from build123d import *

# Parameters (mm, degrees)
SKETCH1_W           = 40
SKETCH1_H           = 29.3
SKETCH1_H_2         = 8.7
BOSS_EXTRUDE1_DEPTH = 20.2
SKETCH2_R           = 2.65
BOSS_EXTRUDE2_DEPTH = 5.2
SKETCH3_W           = 0.446843519
SKETCH3_H           = 1.306192745
SKETCH3_H_2         = 1.306192746
CUT_EXTRUDE1_DEPTH  = 5.2
FILLET1_R           = 3
CHAMFER1_SIZE       = 5
SKETCH4_R           = 6
BOSS_EXTRUDE3_DEPTH = 1
BOSS_EXTRUDE4_DEPTH = 0.5


with BuildPart() as part:
    # Sketch1 → Boss-Extrude1 (new body)
    with BuildSketch(Plane.XY):
        Rectangle(SKETCH1_W, SKETCH1_H)
        Polygon((-27, 14.65), (-20, 14.65), (20, 14.65), (27, 14.65), (27, 17.15), (20, 17.15), (-20, 17.15), (-27, 17.15), align=None)
        with Locations((0, 21.5)):
            Rectangle(SKETCH1_W, SKETCH1_H_2)
    extrude(amount=BOSS_EXTRUDE1_DEPTH)

    # Sketch2 → Boss-Extrude2 (add)
    with BuildSketch(Plane(origin=(0, 25.85, 0), x_dir=(1, 0, 0), z_dir=(0, 1, 0))):
        with Locations((-9.5, -10.1)):
            Circle(SKETCH2_R)
    extrude(amount=BOSS_EXTRUDE2_DEPTH)

    # Sketch3 → Cut-Extrude1 (cut)
    with BuildSketch(Plane(origin=(0, 17.15, 0), x_dir=(1, 0, 0), z_dir=(0, 1, 0))):
        with BuildLine():
            Line((-25.540550997, -5.731244645), (-25.540550997, -4.4250519))
            Line((-25.540550997, -4.4250519), (-25.882669663, -4.4250519))
            ThreePointArc((-25.882669663, -4.4250519), (-25.99986637, -5.076880711), (-25.897769796, -5.731244645))
            Line((-25.897769796, -5.731244645), (-25.540550997, -5.731244645))
        make_face()
        with BuildLine():
            Line((-25.882669663, -4.4250519), (-25.540550997, -4.4250519))
            Line((-25.540550997, -4.4250519), (-25.540550997, -5.731244645))
            Line((-25.540550997, -5.731244645), (-25.897769796, -5.731244645))
            ThreePointArc((-25.897769796, -5.731244645), (-23.680265416, -7.074277031), (-22, -5.1))
            ThreePointArc((-22, -5.1), (-23.657464839, -3.129550898), (-25.882669663, -4.4250519))
        make_face()
        with BuildLine():
            ThreePointArc((-25.897769796, -5.731244645), (-25.99986637, -5.076880711), (-25.882669663, -4.4250519))
            Line((-25.882669663, -4.4250519), (-27.446843519, -4.4250519))
            Line((-27.446843519, -4.4250519), (-27.446843519, -5.731244645))
            Line((-27.446843519, -5.731244645), (-25.897769796, -5.731244645))
        make_face()
        with BuildLine():
            Line((-25.540550997, -15.653096373), (-25.540550997, -14.346903627))
            Line((-25.540550997, -14.346903627), (-25.852794067, -14.346903627))
            ThreePointArc((-25.852794067, -14.346903627), (-25.997198696, -14.994182379), (-25.922000105, -15.653096373))
            Line((-25.922000105, -15.653096373), (-25.540550997, -15.653096373))
        make_face()
        with BuildLine():
            Line((-25.852794067, -14.346903627), (-25.540550997, -14.346903627))
            Line((-25.540550997, -14.346903627), (-25.540550997, -15.653096373))
            Line((-25.540550997, -15.653096373), (-25.922000105, -15.653096373))
            ThreePointArc((-25.922000105, -15.653096373), (-23.720715387, -17.080404026), (-22, -15.1))
            ThreePointArc((-22, -15.1), (-23.616325746, -13.137146448), (-25.852794067, -14.346903627))
        make_face()
        with BuildLine():
            ThreePointArc((-25.922000105, -15.653096373), (-25.997198696, -14.994182379), (-25.852794067, -14.346903627))
            Line((-25.852794067, -14.346903627), (-27.446843519, -14.346903627))
            Line((-27.446843519, -14.346903627), (-27.446843519, -15.653096373))
            Line((-27.446843519, -15.653096373), (-25.922000105, -15.653096373))
        make_face()
        with Locations((27.223421759, -5.078148273)):
            Rectangle(SKETCH3_W, SKETCH3_H)
        with BuildLine():
            ThreePointArc((26, -5.1), (25.974277031, -5.419734584), (25.897769796, -5.731244645))
            Line((25.897769796, -5.731244645), (27, -5.731244645))
            Line((27, -5.731244645), (27, -4.4250519))
            Line((27, -4.4250519), (25.882669663, -4.4250519))
            ThreePointArc((25.882669663, -4.4250519), (25.970449102, -4.757464839), (26, -5.1))
        make_face()
        with BuildLine():
            Line((25.540550997, -4.4250519), (25.540550997, -5.731244645))
            Line((25.540550997, -5.731244645), (25.897769796, -5.731244645))
            ThreePointArc((25.897769796, -5.731244645), (25.974277031, -5.419734584), (26, -5.1))
            ThreePointArc((26, -5.1), (25.970449102, -4.757464839), (25.882669663, -4.4250519))
            Line((25.882669663, -4.4250519), (25.540550997, -4.4250519))
        make_face()
        with BuildLine():
            Line((25.897769796, -5.731244645), (25.540550997, -5.731244645))
            Line((25.540550997, -5.731244645), (25.540550997, -4.4250519))
            Line((25.540550997, -4.4250519), (25.882669663, -4.4250519))
            ThreePointArc((25.882669663, -4.4250519), (22.00013363, -5.123119289), (25.897769796, -5.731244645))
        make_face()
        with Locations((27.223421759, -15)):
            Rectangle(SKETCH3_W, SKETCH3_H_2)
        with BuildLine():
            Line((27, -15.653096373), (27, -14.346903627))
            Line((27, -14.346903627), (25.852794067, -14.346903627))
            ThreePointArc((25.852794067, -14.346903627), (25.962853552, -14.716325746), (26, -15.1))
            ThreePointArc((26, -15.1), (25.980404026, -15.379284613), (25.922000105, -15.653096373))
            Line((25.922000105, -15.653096373), (27, -15.653096373))
        make_face()
        with BuildLine():
            ThreePointArc((26, -15.1), (25.962853552, -14.716325746), (25.852794067, -14.346903627))
            Line((25.852794067, -14.346903627), (25.540550997, -14.346903627))
            Line((25.540550997, -14.346903627), (25.540550997, -15.653096373))
            Line((25.540550997, -15.653096373), (25.922000105, -15.653096373))
            ThreePointArc((25.922000105, -15.653096373), (25.980404026, -15.379284613), (26, -15.1))
        make_face()
        with BuildLine():
            Line((25.540550997, -14.346903627), (25.852794067, -14.346903627))
            ThreePointArc((25.852794067, -14.346903627), (22.002801304, -15.205817621), (25.922000105, -15.653096373))
            Line((25.922000105, -15.653096373), (25.540550997, -15.653096373))
            Line((25.540550997, -15.653096373), (25.540550997, -14.346903627))
        make_face()
    extrude(amount=-CUT_EXTRUDE1_DEPTH, mode=Mode.SUBTRACT)

    # Fillet1
    fillet1_edges = [part.edges().sort_by_distance(p)[0] for p in [
        (-27, 15.9, 0),
        (27, 15.9, 0),
        (27, 15.9, 20.2),
        (-27, 15.9, 20.2),
    ]]
    fillet(fillet1_edges, radius=FILLET1_R)

    # Chamfer1
    chamfer1_edges = [part.edges().sort_by_distance(p)[0] for p in [
        (20, 25.85, 10.1),
    ]]
    chamfer(chamfer1_edges, length=CHAMFER1_SIZE)

    # Sketch4 → Boss-Extrude3 (add)
    with BuildSketch(Plane(origin=(0, 25.85, 0), x_dir=(1, 0, 0), z_dir=(0, 1, 0))):
        with Locations((-9.5, -10.1)):
            Circle(SKETCH4_R)
    extrude(amount=BOSS_EXTRUDE3_DEPTH)

    # Sketch5 → Boss-Extrude4 (add)
    with BuildSketch(Plane(origin=(0, 25.85, 0), x_dir=(1, 0, 0), z_dir=(0, 1, 0))):
        with BuildLine():
            Line((-9.5, -1.789920634), (8.092095239, -1.789920634))
            ThreePointArc((8.092095239, -1.789920634), (9.506308801, -2.375707072), (10.092095239, -3.789920634))
            Line((10.092095239, -3.789920634), (10.092095239, -16.410079366))
            ThreePointArc((10.092095239, -16.410079366), (9.506308801, -17.824292928), (8.092095239, -18.410079366))
            Line((8.092095239, -18.410079366), (-9.5, -18.410079366))
            ThreePointArc((-9.5, -18.410079366), (-17.810079366, -10.1), (-9.5, -1.789920634))
        make_face()
    extrude(amount=BOSS_EXTRUDE4_DEPTH)


solid = part.part
For this review, take the finished solid that the model builds, in its own axes (mm). A direction names the side the tool comes from. Coordinates: 2 decimals unless noted, no trailing zeros. Loops run counter-clockwise (first coordinate to the right, second up) from the corner with the lowest first, then second, coordinate; pieces in that order, holes last. Notation, with made-up numbers: (48.5, -20.5) -> (63.5, -20.5) arc R12 cw to (63.5, -8.5) -> close; hole circle Ø5 at (-35, 69.25). An arc over 180 degrees is marked (long way). Write each question's results on one line, items separated by ' | '.
Q1. Machinability: for faces 1 (the flat face through (-3, 25.85, 1)), 2 (the flat face through (26.4, 15.9, 14.347)), 3 (the flat face through (-24, 14.65, 10)), 4 (the flat face through (-23, 17.15, 10)), 5 (the flat face through (20, 0, 10)), which of the approach directions +Z, -Z, +X, -X, +Y, -Y give a long, thin tool a straight path to every point of the face, cutting with its end or side? Answer none if there is none.
Taken from the geometry:
face 1: +Y | face 2: +X, +Y, -Y | face 3: +Z, -Z, -X, -Y | face 4: +Z, -Z, -X, +Y | face 5: +Z, -Z, +X, -Y
Q2. Add section C-C, the plane x = 16. State the section outline as (y, z) points, then the cut area to 3 significant figures.
Taken from the geometry:
outline: (-14.65, 0) -> (24.85, 0) -> (24.85, 20.2) -> (-14.65, 20.2) -> close | area: 798 mm²
Q3. Add section B-B, the plane y = 9. State the section outline as (x, z) points, then the cut area to 3 significant figures.
Taken from the geometry:
outline: (-20, 0) -> (20, 0) -> (20, 20.2) -> (-20, 20.2) -> close | area: 808 mm²
Q4. To check wall thickness, follow line 1 along Z through (x, y) = (24, 16); line 2 along X through (y, z) = (15.65, 5.1); line 3 along Y through (x, z) = (5.5, 13). State the ranges of each line that lie inside material, in increasing order. Write a range as [from, to].
Taken from the geometry:
line 1: [0, 3.1], [7.1, 13.1], [17.1, 20.2] | line 2: [-22, 22] | line 3: [-14.65, 26.35]
Q5. For pin 1 Ø0.6 at (x, y) = (-26, 15.5) entering from +Z; pin 2 Ø3.5 at (x, z) = (24, 7.5) entering from -Y; pin 3 Ø3.5 at (x, z) = (22.5, 8) entering from +Y, all flat-tipped, find the tip position at first contact; note any pin that passes through.
Taken from the geometry:
pin 1: z = 19.67 | pin 2: y = 14.65 | pin 3: y = 17.15
Q6. Add section A-A, the plane x = -8.5. State the section outline as (y, z) points.
Taken from the geometry:
outline: (-14.65, 0) -> (25.85, 0) -> (25.85, 1.79) -> (26.35, 1.79) -> (26.35, 4.18) -> (26.85, 4.18) -> (26.85, 7.65) -> (31.05, 7.65) -> (31.05, 12.55) -> (26.85, 12.55) -> (26.85, 16.02) -> (26.35, 16.02) -> (26.35, 18.41) -> (25.85, 18.41) -> (25.85, 20.2) -> (-14.65, 20.2) -> close
Q7. Mouldability with a two-part tool opening along X and no side actions: class faces 6 (the flat face through (27, 16, 16)), 7 (the cylindrical face through (-26.1, 15.88, 0.86)), 8 (the cylindrical face through (22, 15.9, 15.1)), 9 (the flat face through (24, 17.15, 10)) as +X half, -X half, draft (parallel to the pull), parting line (faces both ways), or undercut.
Taken from the geometry:
face 6: +X half | face 7: -X half | face 8: undercut | face 9: draft
